Part model, mm, in its own coordinate system. Face numbers are marked on the shaded views. Give positions to 0.01 mm unless a question says otherwise; leave off trailing zeros. Write each loop counter-clockwise with the first axis right and the second up, starting at its lowest first coordinate (ties: lowest second). Pieces come first, ordered by that corner, then holes. Notation, with made-up numbers: M 78.5,12.25 L 135.5,12.25 A29 cw 135.5,42.25 Z; hole C 78,48 d4. An arc over 180 degrees is marked long. Write item = value, one per line. Start each with the question number.
from build123d import *

# Parameters (mm, degrees)
SKETCH1_W           = 12
SKETCH1_H           = 12
BOSS_EXTRUDE1_DEPTH = 4.3
SKETCH2_W           = 3.8
SKETCH2_H           = 3.8
BOSS_EXTRUDE2_DEPTH = 3
SKETCH3_W           = 106
SKETCH3_H           = 36
BOSS_EXTRUDE3_DEPTH = 1.6
SKETCH4_W           = 12
SKETCH4_H           = 12
BOSS_EXTRUDE4_DEPTH = 4.3
SKETCH5_W           = 3.8
SKETCH5_H           = 3.8
BOSS_EXTRUDE5_DEPTH = 3


with BuildPart() as part:
    # Sketch1 → Boss-Extrude1 (new body)
    with BuildSketch(Plane(origin=(0, 0, 0), x_dir=(1, 0, 0), z_dir=(0, 1, 0))):
        with Locations((6, 6)):
            Rectangle(SKETCH1_W, SKETCH1_H)
    extrude(amount=BOSS_EXTRUDE1_DEPTH)

    # Sketch2 → Boss-Extrude2 (add)
    with BuildSketch(Plane(origin=(0, 4.3, 0), x_dir=(1, 0, 0), z_dir=(0, 1, 0))):
        with Locations((6, 6)):
            Rectangle(SKETCH2_W, SKETCH2_H)
    extrude(amount=BOSS_EXTRUDE2_DEPTH)

    # Sketch3 → Boss-Extrude3 (add)
    with BuildSketch(Plane.XZ):
        with Locations((41, -6)):
            Rectangle(SKETCH3_W, SKETCH3_H)
    extrude(amount=BOSS_EXTRUDE3_DEPTH)

    # Sketch4 → Boss-Extrude4 (add)
    with BuildSketch(Plane(origin=(0, 0, 0), x_dir=(1, 0, 0), z_dir=(0, 1, 0))):
        with Locations((41, 6)):
            Rectangle(SKETCH4_W, SKETCH4_H)
        with Locations((76, 6)):
            Rectangle(SKETCH4_W, SKETCH4_H)
    extrude(amount=BOSS_EXTRUDE4_DEPTH)

    # Sketch5 → Boss-Extrude5 (add)
    with BuildSketch(Plane(origin=(0, 4.3, 0), x_dir=(1, 0, 0), z_dir=(0, 1, 0))):
        with Locations((41, 6)):
            Rectangle(SKETCH5_W, SKETCH5_H)
        with Locations((76, 6)):
            Rectangle(SKETCH5_W, SKETCH5_H)
    extrude(amount=BOSS_EXTRUDE5_DEPTH)


solid = part.part
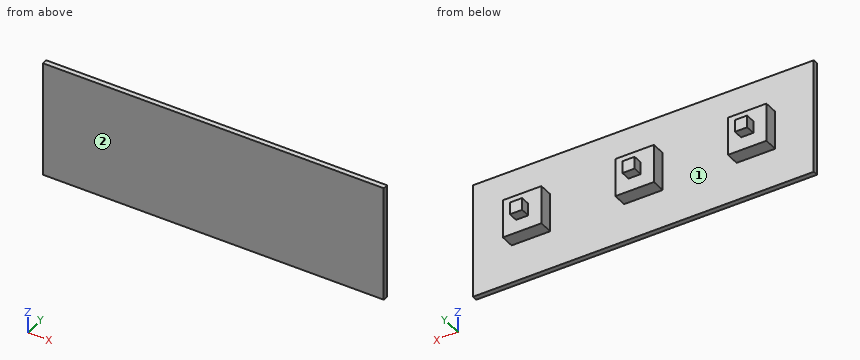
Q1. Slice it at B-B (x = 36.5). Give the cut face in (y, z), and give its area (3 significant figures).
Q2. Slice it at A-A (y = 5.75). Give the cut face in (x, z), and give its area (3 significant figures).
Q3. Drop flat-ended pins along their axis: P1, Ø3.5, axis at y = 2.5, z = -4, coming from the +X side; P2, Ø0.9, axis at x = 75.5, y = 6, coming from the +Z side; P3, Ø3.5, axis at x = 73.5, y = 2.5, coming from the -Z side. Give the stop position or say it passes through.
Q4. Probe line 1 along X through (y, z) = (3, -6.5); line 2 along Y through (x, z) = (61, -0.5); line 3 along Y through (x, z) = (37.5, -2). List the from-to ranges inside material, lowest first.
Q5. Slice it at D-D (y = 1). Give the cut face in (x, z), and give its area (3 significant figures).
Q6. Slice it at C-C (z = -9). Give the cut face in (x, y).
Q7. Two-plate mould, pull along X, no slides. Class the marked faces 1 and 2: +X half, -X half, draft (parallel to the pull), parting line (faces both ways), or undercut.
Working result:
q1.outline = M -1.6,-24 L 0,-24 L 0,-12 L 4.3,-12 L 4.3,0 L 0,0 L 0,12 L -1.6,12 Z
q1.area = 109 mm2
q2.outline = M 4.1,-7.9 L 7.9,-7.9 L 7.9,-4.1 L 4.1,-4.1 Z; M 39.1,-7.9 L 42.9,-7.9 L 42.9,-4.1 L 39.1,-4.1 Z; M 74.1,-7.9 L 77.9,-7.9 L 77.9,-4.1 L 74.1,-4.1 Z
q2.area = 43.3 mm2
q3.P1 = 82
q3.P2 = -4.1
q3.P3 = -12
q4.line_1 = 0 to 12, 35 to 47, 70 to 82
q4.line_2 = -1.6 to 0
q4.line_3 = -1.6 to 4.3
q5.outline = M 0,-12 L 12,-12 L 12,0 L 0,0 Z; M 35,-12 L 47,-12 L 47,0 L 35,0 Z; M 70,-12 L 82,-12 L 82,0 L 70,0 Z
q5.area = 432 mm2
q6.outline = M -12,-1.6 L 94,-1.6 L 94,0 L 82,0 L 82,4.3 L 70,4.3 L 70,0 L 47,0 L 47,4.3 L 35,4.3 L 35,0 L 12,0 L 12,4.3 L 0,4.3 L 0,0 L -12,0 Z
q7.face_1 = undercut
q7.face_2 = draft
